Can you work these out from the drawing? Everything is in mm from the part's minimum corner. A direction names the side the tool comes from. Coordinates: 2 decimals unless noted, no trailing zeros. Loops run counter-clockwise (first coordinate to the right, second up) from the corner with the lowest first, then second, coordinate; pieces in that order, holes last. Notation, with made-up numbers: (42, -20.5) - (77, -20.5) arc R14 cw to (77, -12.5) - close; hole circle Ø1 at (-3.75, -37). An arc over 180 degrees is marked (long way). Put each result on its own line as item: value. Start each with the question number.
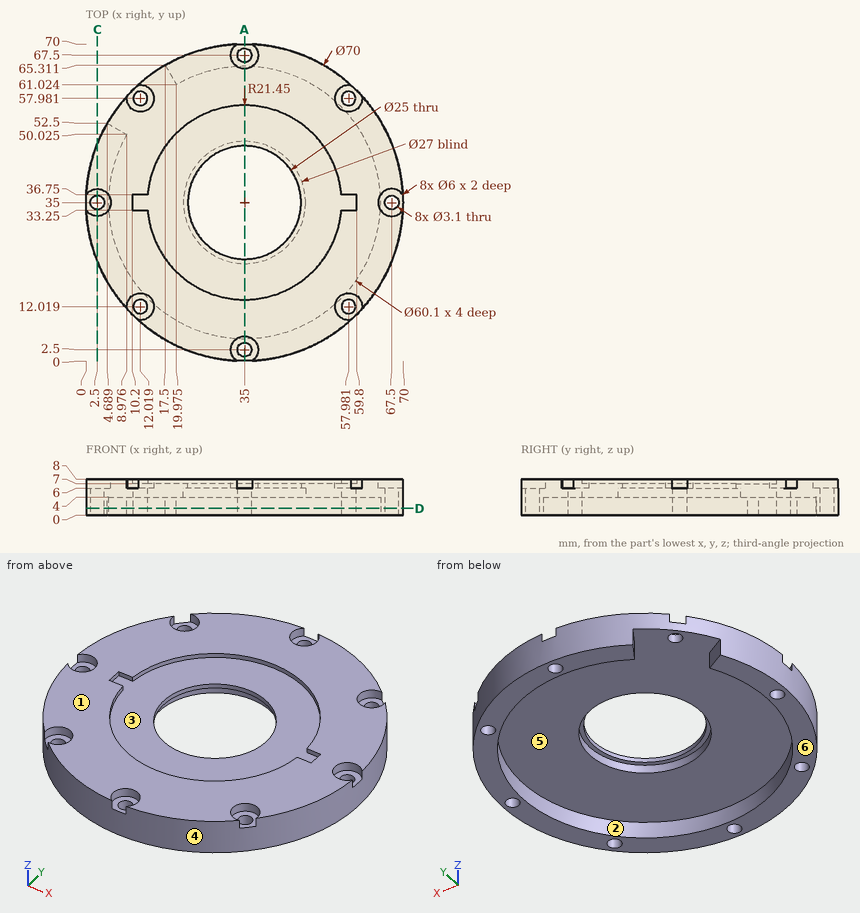
(1) I want a section at C-C on x = 2.5. List the corners of the cut face in (y, z) for me.
(2) For pin 1 Ø1 at (x, z) = (56, 5.5) entering from -Y; pin 2 Ø5 at (x, y) = (12.02, 12.02) entering from +Z; pin 3 Ø8 at (x, y) = (21.5, 27.5) entering from +Z, each with a flat end and sliding along its axis, tell me the tip position at first contact or that it passes through.
(3) I want a section at D-D on z = 1.5. List the corners of the cut face in (x, y) for me (3 decimals).
(4) I want a section at A-A on x = 35. Count the separate pieces of the cut face and the enclosed holes in it, and give its area (4 significant figures).
(5) I need wall thicknesses on L1, parallel to Y at x = 35, z = 3.7; L2, parallel to X at y = 35, z = 7.5; L3, parallel to Z at x = 42, y = 18.5. Which ranges of each line are inside material? Lowest first, please. Write a range as [from, to].
(6) If we mould it in two halves opening along Y, with no side actions, what happens to the marked faces 4, 5 and 6? For each: pulls with the +Y half, pulls with the -Y half, needs draft (parallel to the pull), parting line crosses it, or undercut.
(7) Which directions (+Z, -Z, +X, -X, +Y, -Y) give clear straight access to the entire face, cutting with the end or side of a thin tool? Please do the marked faces 1, 2 and 3.
Answer sheet:
1. outline: (22.01, 0) - (33.45, 0) - (33.45, 6) - (32, 6) - (32, 8) - (22.01, 8) - close; (36.55, 0) - (47.99, 0) - (47.99, 8) - (38, 8) - (38, 6) - (36.55, 6) - close
2. pin 1: stops at y = 6.63
2. pin 2: stops at z = 6
2. pin 3: stops at z = 7
3. outline: (4.689, 52.5) arc R35 ccw (long way) to (17.5, 65.311) - (19.975, 61.024) arc R30.05 cw (long way) to (8.976, 50.025) - close; hole circle Ø3.1 at (2.5, 35); hole circle Ø3.1 at (12.019, 12.019); hole circle Ø3.1 at (35, 2.5); hole circle Ø3.1 at (35, 67.5); hole circle Ø3.1 at (57.981, 12.019); hole circle Ø3.1 at (57.981, 57.981); hole circle Ø3.1 at (67.5, 35)
4. separate pieces: 4
4. enclosed holes: 0
4. area: 138.5 mm^2
5. L1: y = [0, 0.95], [4.05, 4.95], [65.05, 65.95], [69.05, 70]
5. L2: x = [5.5, 10.2], [59.8, 64.5]
5. L3: z = [4, 7]
6. face 4: parting line crosses it
6. face 5: undercut
6. face 6: needs draft
7. face 1: +Z, +X, -X, +Y, -Y
7. face 2: -Z
7. face 3: +Z
